from build123d import *

# Parameters (mm, degrees)
EXTRU_MINCE1_DEPTH      = 103.5
ESQUISSE2_R             = 1.5
ENL_V_MAT_EXTRU_1_DEPTH = 3
ESQUISSE3_R             = 1.5
ENL_V_MAT_EXTRU_2_DEPTH = 3


with BuildPart() as part:
    # Esquisse1 → Extru.-Mince1 (new, symmetric)
    with BuildSketch(Plane.XY):
        Polygon((0, 10), (0, 0), (10, 0), (10, 1), (1, 1), (1, 10), align=None)
    extrude(amount=EXTRU_MINCE1_DEPTH, both=True)

    # Esquisse2 → Enlèv. mat.-Extru.1 (cut)
    with BuildSketch(Plane(origin=(0, 1, 0), x_dir=(1, 0, 0), z_dir=(0, 1, 0))):
        with Locations(Location((6, 56.3, 0), (0, 0, 270))):
            Circle(ESQUISSE2_R)
        with Locations(Location((6, -56.3, 0), (0, 0, 270))):
            Circle(ESQUISSE2_R)
    extrude(amount=-ENL_V_MAT_EXTRU_1_DEPTH, mode=Mode.SUBTRACT)

    # Esquisse3 → Enlèv. mat.-Extru.2 (cut)
    with BuildSketch(Plane(origin=(1, 0, 0), x_dir=(0, 0, -1), z_dir=(1, 0, 0))):
        with Locations(Location((-99, 5.5, 0), (0, 0, 90))):
            Circle(ESQUISSE3_R)
        with Locations(Location((99, 5.5, 0), (0, 0, 90))):
            Circle(ESQUISSE3_R)
    extrude(amount=-ENL_V_MAT_EXTRU_2_DEPTH, mode=Mode.SUBTRACT)


solid = part.part
Work out the finished part from the listing and answer in its coordinate system (mm). A direction names the side the tool comes from. Coordinates: 2 decimals unless noted, no trailing zeros. Order: outer loops, then holes, each group sorted by start corner. A loop starts at its lowest first (then second) coordinate and runs counter-clockwise, first axis right, second up. Notation, with made-up numbers: (-30, -1) - (12, -1) arc R7 ccw to (12, 12) - close; hole circle Ø2 at (-3, 17). An arc over 180 degrees is marked (long way). Put each result on its own line as item: value. Start each with the question number.
1) Find section B-B (z = -29). Give the vertices of the cut face in (x, y).
2) Find the intervals of material crossed by line 1 (Z direction, x = 0.7, y = 5.5); line 2 (X direction, y = 0.65, z = -56.3); line 3 (Y direction, x = 0.6, z = -99), in increasing order. Write a range as from..to.
3) Flat-ended cylindrical pins translate along their axes: pin 1 (2.5 mm diameter, centred on y = 5.5, z = -99, fed in from -X); pin 2 (1 mm diameter, centred on x = 6.5, z = 0.5, fed in from +Y); pin 3 (2 mm diameter, centred on y = 6.5, z = -46.5, fed in from +X). Find the tip coordinate at first contact, or state that the pin passes through.
4) For faces 1 (the flat face through (5, 0, 1)), 2 (the flat face through (1, 5, 1)), determine the directions among +Z, -Z, +X, -X, +Y, -Y from which every point of the face is accessible in a straight line to the end or side of a thin tool.
5) Find section C-C (y = 2.5). Give the vertices of the cut face in (x, z), plus the area to 3 significant figures.
6) Find section A-A (x = 6). Give the vertices of the cut face in (y, z).
Results list:
1. outline: (0, 0) - (10, 0) - (10, 1) - (1, 1) - (1, 10) - (0, 10) - close
2. line 1: z = -103.5..-100.5, -97.5..97.5, 100.5..103.5
2. line 2: x = 0..4.5, 7.5..10
2. line 3: y = 0..4, 7..10
3. pin 1: passes through
3. pin 2: stops at y = 1
3. pin 3: stops at x = 1
4. face 1: +Z, -Z, +X, -X, -Y
4. face 2: +Z, -Z, +X, +Y
5. outline: (0, -103.5) - (1, -103.5) - (1, 103.5) - (0, 103.5) - close
5. area: 207 mm^2
6. outline: (0, -103.5) - (1, -103.5) - (1, -57.8) - (0, -57.8) - close; (0, -54.8) - (1, -54.8) - (1, 54.8) - (0, 54.8) - close; (0, 57.8) - (1, 57.8) - (1, 103.5) - (0, 103.5) - close
